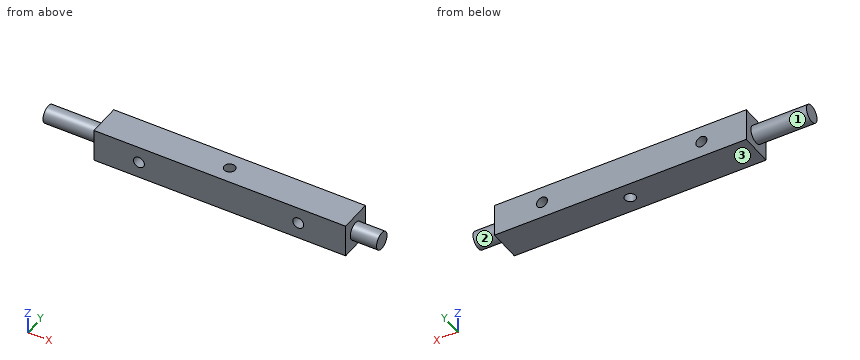
```python
from build123d import *

# Parameters (mm, degrees)
CROQUIS1_W              = 15
CROQUIS1_H              = 15
SALIENTE_EXTRUIR1_DEPTH = 57.5
CROQUIS2_R              = 2.5
CORTAR_EXTRUIR1_DEPTH   = 60.895742754
CROQUIS3_R              = 2.5
CORTAR_EXTRUIR2_DEPTH   = 60.895742754
CROQUIS4_R              = 4
SALIENTE_EXTRUIR2_DEPTH = 25.4
CROQUIS5_R              = 3.976569184
SALIENTE_EXTRUIR3_DEPTH = 12


with BuildPart() as part:
    # Croquis1 → Saliente-Extruir1 (new, symmetric)
    with BuildSketch(Plane(origin=(0, 0, 0), x_dir=(0, 0, -1), z_dir=(1, 0, 0))):
        Rectangle(CROQUIS1_W, CROQUIS1_H)
    extrude(amount=SALIENTE_EXTRUIR1_DEPTH, both=True)

    # Croquis2 → Cortar-Extruir1 (cut, through all)
    with BuildSketch(Plane.XY.offset(7.5)):
        Circle(CROQUIS2_R)
    extrude(amount=-CORTAR_EXTRUIR1_DEPTH, mode=Mode.SUBTRACT)

    # Croquis3 → Cortar-Extruir2 (cut, through all)
    with BuildSketch(Plane(origin=(0, 7.5, 0), x_dir=(1, 0, 0), z_dir=(0, 1, 0))):
        with Locations(Location((-36.974332256, 0, 0), (0, 0, 270))):
            Circle(CROQUIS3_R)
        with Locations(Location((35.85631789, 0, 0), (0, 0, 270))):
            Circle(CROQUIS3_R)
    extrude(amount=-CORTAR_EXTRUIR2_DEPTH, mode=Mode.SUBTRACT)

    # Croquis4 → Saliente-Extruir2 (add)
    with BuildSketch(Plane.ZY.offset(57.5)):
        with Locations(Location((0, 0, 0), (0, 0, 180))):
            Circle(CROQUIS4_R)
    extrude(amount=SALIENTE_EXTRUIR2_DEPTH)

    # Croquis5 → Saliente-Extruir3 (add)
    with BuildSketch(Plane(origin=(57.5, 0, 0), x_dir=(0, 0, -1), z_dir=(1, 0, 0))):
        Circle(CROQUIS5_R)
    extrude(amount=SALIENTE_EXTRUIR3_DEPTH)


solid = part.part
```
Source: CAD feature listing. Evaluate the final solid. Frame: model axes, mm. Face numbers are marked on the shaded views. A direction names the side the tool comes from. Round coordinates to 2 decimals unless told otherwise and drop trailing zeros. Loops run counter-clockwise (first coordinate to the right, second up) from the corner with the lowest first, then second, coordinate; pieces in that order, holes last.
1. Section query C-C on x = 0. Output: boundary loops of the cut face in (y, z).
2. Ray query, L1, parallel to X at y = 4.75, z = 0; L2, parallel to X at y = 2.75, z = 0; L3, parallel to X at y = -0.25, z = 0. Return the intervals inside material, ascending.
3. Section query B-B on y = 0. Output: boundary loops of the cut face in (x, z).
4. Contact query for a flat-ended pin moving along its axis: pin 1 (4 mm diameter, centred on y = 5, z = 4.5, fed in from -X). Output: stop coordinate, or through.
5. Access query for the marked faces 1, 2 and 3. Directions: +Z, -Z, +X, -X, +Y, -Y. A direction counts if a zero-diameter tool reaches every point of the face in a straight line with its end or side. Return the directions, or none.
6. Section query A-A on z = 0. Output: boundary loops of the cut face in (x, y), and give its area (3 significant figures).
7. Section query D-D on z = -6. Output: boundary loops of the cut face in (x, y), and give its area (3 significant figures).
Answers below:
1. outline: (-7.5, -7.5) - (-2.5, -7.5) - (-2.5, 7.5) - (-7.5, 7.5) - close; (2.5, -7.5) - (7.5, -7.5) - (7.5, 7.5) - (2.5, 7.5) - close
2. L1: x = -57.5 to -39.47, -34.47 to 33.36, 38.36 to 57.5
2. L2: x = -82.9 to -39.47, -34.47 to 33.36, 38.36 to 69.5
2. L3: x = -82.9 to -39.47, -34.47 to -2.49, 2.49 to 33.36, 38.36 to 69.5
3. outline: (-82.9, -4) - (-57.5, -4) - (-57.5, -7.5) - (-2.5, -7.5) - (-2.5, 7.5) - (-57.5, 7.5) - (-57.5, 4) - (-82.9, 4) - close; (2.5, -7.5) - (57.5, -7.5) - (57.5, -3.98) - (69.5, -3.98) - (69.5, 3.98) - (57.5, 3.98) - (57.5, 7.5) - (2.5, 7.5) - close; hole circle Ø5 at (-36.97, 0); hole circle Ø5 at (35.86, 0)
4. pin 1: stops at x = -57.5
5. face 1: -X
5. face 2: +X
5. face 3: -Z, +X, -X, +Y, -Y
6. outline: (-82.9, -4) - (-57.5, -4) - (-57.5, -7.5) - (-39.47, -7.5) - (-39.47, 7.5) - (-57.5, 7.5) - (-57.5, 4) - (-82.9, 4) - close; (-34.47, -7.5) - (33.36, -7.5) - (33.36, 7.5) - (-34.47, 7.5) - close; (38.36, -7.5) - (57.5, -7.5) - (57.5, -3.98) - (69.5, -3.98) - (69.5, 3.98) - (57.5, 3.98) - (57.5, 7.5) - (38.36, 7.5) - close; hole circle Ø5 at (0, 0)
6. area: 1,850 mm2
7. outline: (-57.5, -7.5) - (57.5, -7.5) - (57.5, 7.5) - (-57.5, 7.5) - close; hole circle Ø5 at (0, 0)
7. area: 1,710 mm2
